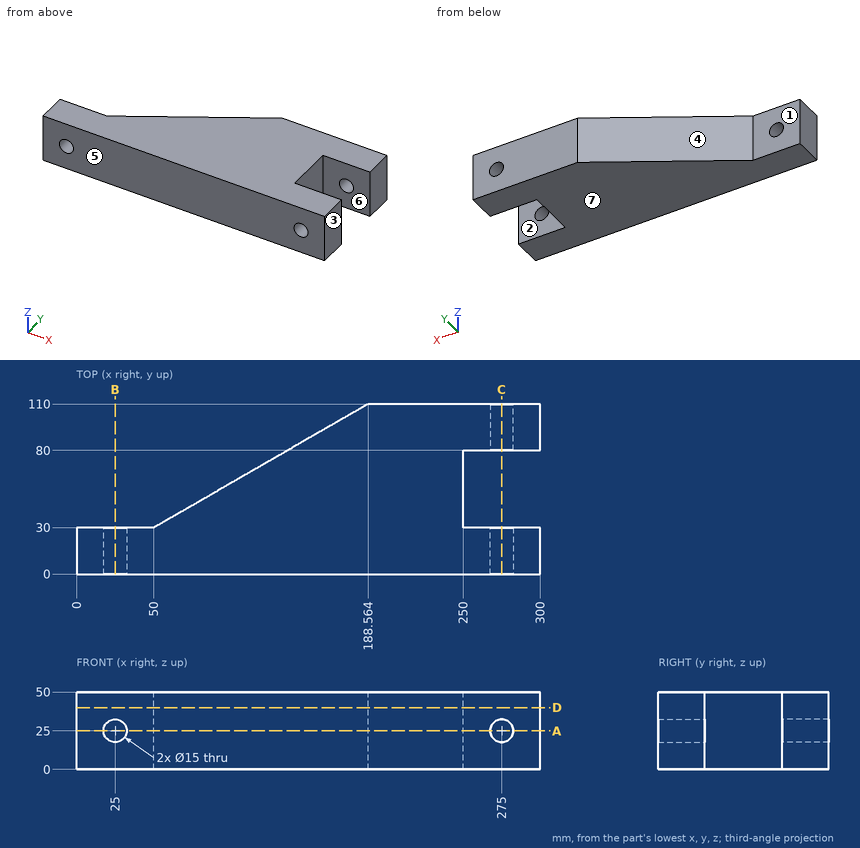
Geometry: see drawing. Coordinates: mm, zero at the bounding-box minimum. A direction names the side the tool comes from. Give positions to 0.01 mm unless a question says otherwise; leave off trailing zeros. Write each loop counter-clockwise with the first axis right and the second up, starting at its lowest first coordinate (ties: lowest second). Pieces come first, ordered by that corner, then holes. Notation, with made-up numbers: M 28,84 L 59,84 A10 ccw 59,95 Z; hole C 80,53 d1. An arc over 180 degrees is marked long. Answer in a Markdown table with one row per item. Add a question column.
(1) Reachability of the marked faces 1, 2 and 3 from +Z, -Z, +X, -X, +Y, -Y: full face, straight path, thin tool, end or side. Return the list, or none.
(2) Section A-A on z = 25. Return loops of the section in (x, y), and give its area (3 significant figures).
(3) First-contact query: pin 1 (2 mm diameter, centred on x = 166, z = 5, fed in from +Y); pin 2 (3 mm diameter, centred on y = 34.5, z = 15, fed in from -X). Flat tips, straight axial feed; report the tip coordinate or a pass-through.
(4) Ray query, line 1 (X direction, y = 19.25, z = 25); line 2 (Z direction, x = 275, y = 23.25); line 3 (Y direction, x = 15, z = 11.5). Return the intervals inside material, ascending.
(5) Mould query, pull axis Y, two halves, no side actions, for the marked faces 4, 5, 6 and 7. Classes: +Y half, -Y half, draft (parallel to the pull), parting line (faces both ways), or undercut.
(6) Section D-D on z = 40. Return loops of the section in (x, y).
(7) Section C-C on x = 275. Return loops of the section in (y, z), and give its area (3 significant figures).
(8) Section B-B on x = 25. Return loops of the section in (y, z).
Result set:
| question | item | result |
|---|---|---|
| 1 | face 1 | +Z, -Z, -X, +Y |
| 1 | face 2 | +Z, -Z, +X |
| 1 | face 3 | +Z, -Z, +X, +Y, -Y |
| 2 | outline | M 0,0 L 17.5,0 L 17.5,30 L 0,30 Z; M 32.5,0 L 267.5,0 L 267.5,30 L 250,30 L 250,80 L 267.5,80 L 267.5,110 L 188.56,110 L 50,30 L 32.5,30 Z; M 282.5,0 L 300,0 L 300,30 L 282.5,30 Z; M 282.5,80 L 300,80 L 300,110 L 282.5,110 Z |
| 2 | area | 19,600 mm^2 |
| 3 | pin 1 | stops at y = 97.55 |
| 3 | pin 2 | stops at x = 55.2 |
| 4 | line 1 | x = 0 to 17.5, 32.5 to 267.5, 282.5 to 300 |
| 4 | line 2 | z = 0 to 17.5, 32.5 to 50 |
| 4 | line 3 | y = 0 to 30 |
| 5 | face 4 | +Y half |
| 5 | face 5 | -Y half |
| 5 | face 6 | undercut |
| 5 | face 7 | draft |
| 6 | outline | M 0,0 L 300,0 L 300,30 L 250,30 L 250,80 L 300,80 L 300,110 L 188.56,110 L 50,30 L 0,30 Z |
| 7 | outline | M 0,0 L 30,0 L 30,17.5 L 0,17.5 Z; M 0,32.5 L 30,32.5 L 30,50 L 0,50 Z; M 80,0 L 110,0 L 110,17.5 L 80,17.5 Z; M 80,32.5 L 110,32.5 L 110,50 L 80,50 Z |
| 7 | area | 2,100 mm^2 |
| 8 | outline | M 0,0 L 30,0 L 30,17.5 L 0,17.5 Z; M 0,32.5 L 30,32.5 L 30,50 L 0,50 Z |
